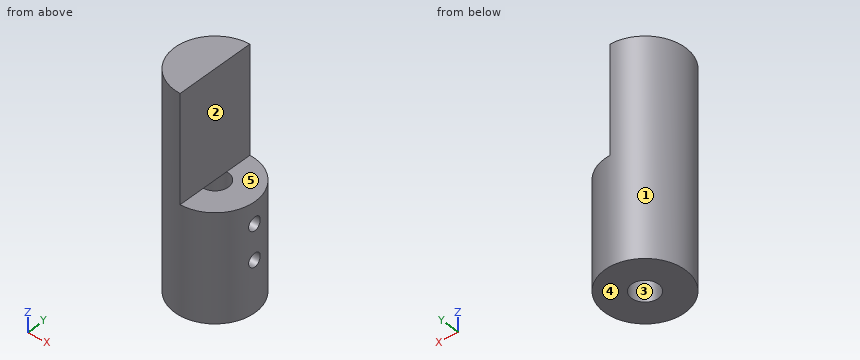
from build123d import *

# Parameters (mm, degrees)
F0_R     = 7.5
F1_DEPTH = 40
F2_W     = 31.443845
F2_H     = 29.544295
F3_DEPTH = 20
F4_R     = 2.5
F5_DEPTH = 20
F6_R     = 1.25
F7_DEPTH = 15


with BuildPart() as f1:
    # F0 (on Top) → F1 (new body)
    with BuildSketch(Plane.XY):
        Circle(F0_R)
    extrude(amount=F1_DEPTH)

    # F2 (on face) → F3 (cut)
    with BuildSketch(Plane.XY.offset(40)):
        with Locations((15.721922, -7.272147)):
            Rectangle(F2_W, F2_H)
    extrude(amount=-F3_DEPTH, mode=Mode.SUBTRACT)

    # F4 (on face) → F5 (cut)
    with BuildSketch(Plane(origin=(0, 0, 0), x_dir=(1, 0, 0), z_dir=(0, 0, -1))):
        Circle(F4_R)
    extrude(amount=-F5_DEPTH, mode=Mode.SUBTRACT)

    # F6 (on face) → F7 (cut)
    with BuildSketch(Plane.YZ):
        with Locations((0, 16)):
            Circle(F6_R)
        with Locations((0, 9.5)):
            Circle(F6_R)
    extrude(amount=F7_DEPTH, mode=Mode.SUBTRACT)


solid = f1.part
Verification items for the finished model (mm, model axes). Face numbers are marked on the shaded views. A direction names the side the tool comes from. Round coordinates to 2 decimals unless told otherwise and drop trailing zeros. Order: outer loops, then holes, each group sorted by start corner. A loop starts at its lowest first (then second) coordinate and runs counter-clockwise, first axis right, second up. Notation, with made-up numbers: (68, -9) -> (109, -9) arc R16 ccw to (109, -4) -> close; hole circle Ø11 at (9, -18). An arc over 180 degrees is marked (long way). Put each result on its own line as item: value.
1) Section check D-D (z = 7). Record the cut outline in (x, y), then the cut area to 3 significant figures.
Final values:
outline: circle Ø15 at (0, 0); hole circle Ø5 at (0, 0)
area: 157 mm^2
2) Section check A-A (y = 0). Record the cut outline in (x, z), then the cut area to 3 significant figures.
Final values:
outline: (-7.5, 0) -> (-2.5, 0) -> (-2.5, 20) -> (0, 20) -> (0, 40) -> (-7.5, 40) -> close; (2.5, 0) -> (7.5, 0) -> (7.5, 8.25) -> (2.5, 8.25) -> close; (2.5, 10.75) -> (7.5, 10.75) -> (7.5, 14.75) -> (2.5, 14.75) -> close; (2.5, 17.25) -> (7.5, 17.25) -> (7.5, 20) -> (2.5, 20) -> close
area: 325 mm^2
3) Section check B-B (x = 1.5). Record the cut outline in (y, z), then the cut area to 3 significant figures.
Final values:
outline: (-7.35, 0) -> (-2, 0) -> (-2, 20) -> (-7.35, 20) -> close; (2, 0) -> (7.35, 0) -> (7.35, 20) -> (2, 20) -> close
area: 214 mm^2
4) Section check C-C (x = 6.5). Record the cut outline in (y, z), then the cut area to 3 significant figures.
Final values:
outline: (-3.74, 0) -> (3.74, 0) -> (3.74, 20) -> (-3.74, 20) -> close; hole circle Ø2.5 at (0, 9.5); hole circle Ø2.5 at (0, 16)
area: 140 mm^2
5) Material ranges on line 1 (Z direction, x = 4.45, y = 0); line 2 (X direction, y = 0, z = 13.25), recorded low to high.
Final values:
line 1: z = 0 to 8.25, 10.75 to 14.75, 17.25 to 20
line 2: x = -7.5 to -2.5, 2.5 to 7.5
6) Depth check by flat-ended pin: pin 1 (4.5 mm diameter, centred on y = -3, z = 26, fed in from +X); pin 2 (1.5 mm diameter, centred on x = -1.5, z = 21, fed in from +Y); pin 3 (5 mm diameter, centred on y = 3, z = 11.5, fed in from +X). Enter the tip coordinate at first touch or a pass-through.
Final values:
pin 1: stops at x = 0
pin 2: stops at y = 7.46
pin 3: stops at x = 7.48
7) Set-up check for the marked faces 4 and 5: record each of +Z, -Z, +X, -X, +Y, -Y from which the full face is reachable in a straight line by a thin tool's end or side.
Final values:
face 4: -Z, +X, -X, +Y, -Y
face 5: +Z, +X, +Y, -Y
8) Mould release check, pull along Y, two halves, no side actions. Record for the marked faces 1, 2 and 3: +Y half, -Y half, draft (parallel to the pull), parting line (faces both ways), or undercut.
Final values:
face 1: parting line
face 2: draft
face 3: undercut
